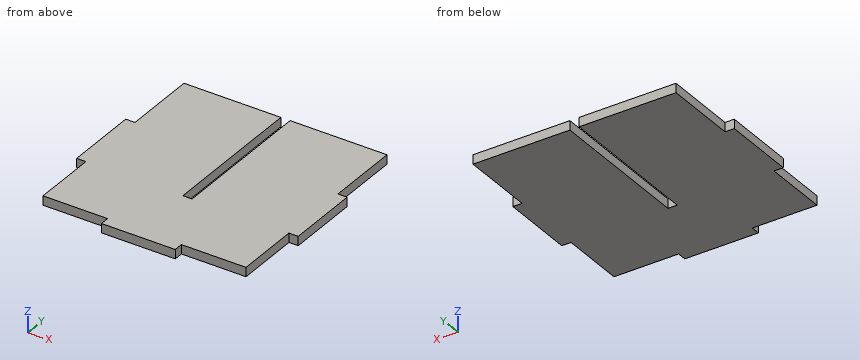
from build123d import *

# Parameters (mm, degrees)
F0_W     = 3.175
F0_H     = 25.4
F0_W_2   = 25.4
F0_H_2   = 3.175
F1_DEPTH = 3.175


with BuildPart() as f1:
    # F0 (on Top) → F1 (new body)
    with BuildSketch(Plane.XY):
        Polygon((34.925, -47.625), (34.925, -25.4), (1.5875, -25.4), (-1.5875, -25.4), (-34.925, -25.4), (-34.925, -47.625), (-12.7, -47.625), (12.7, -47.625), align=None)
        Polygon((1.5875, -25.4), (34.925, -25.4), (34.925, 0), (34.925, 25.4), (1.5875, 25.4), align=None)
        with Locations((36.5125, -12.7)):
            Rectangle(F0_W, F0_H)
        Polygon((-34.925, -25.4), (-1.5875, -25.4), (-1.5875, 25.4), (-34.925, 25.4), (-34.925, 0), align=None)
        with Locations((0, -49.2125)):
            Rectangle(F0_W_2, F0_H_2)
        with Locations((-36.5125, -12.7)):
            Rectangle(F0_W, F0_H)
    extrude(amount=F1_DEPTH)


solid = f1.part
For this review, take the finished solid that the model builds, in its own axes (mm). Give positions to 0.01 mm unless a question says otherwise; leave off trailing zeros. Loops run counter-clockwise (first coordinate to the right, second up) from the corner with the lowest first, then second, coordinate; pieces in that order, holes last. Notation, with made-up numbers: M -25.75,-35.5 L 3.25,-35.5 A11 ccw 3.25,-30.5 Z; hole C 8,-9 d8. An arc over 180 degrees is marked long. Put each result on its own line as item: value. Start each with the question number.
(1) Add section D-D, the plane x = 0. Write out the cut boundary in (y, z) (3 decimals), then the cut area to 3 significant figures.
(2) For pin 1 (1.6 mm diameter, centred on x = 36.5, z = 1.5, fed in from -Y); pin 2 (1.5 mm diameter, centred on y = 1, z = 1.5, fed in from -X) (3 decimals); pin 3 (1.6 mm diameter, centred on y = -50, z = 2.5, fed in from +X); pin 4 (1 mm diameter, centred on x = -25.5, y = -27, fed in from -Z), all flat-tipped, find the tip position at first contact; note any pin that passes through.
(3) Wall thickness on L1, parallel to X at y = 14, z = 2.05 (1 decimal); L2, parallel to X at y = -19, z = 0.5; L3, parallel to Y at x = -33, z = 0.2 (3 decimals): over which ranges is each line inside the solid? List them lowest first.
(4) Add section A-A, the plane y = -6. Write out the cut boundary in (x, z) (1 decimal), then the cut area to 3 significant figures.
(5) Add section C-C, the plane y = 3. Write out the cut boundary in (x, z) (1 decimal).
(6) Add section B-B, the plane z = 0.8. Write out the cut boundary in (x, y) (1 decimal), then the cut area to 3 significant figures.
Result:
1. outline: M -50.8,0 L -25.4,0 L -25.4,3.175 L -50.8,3.175 Z
1. area: 80.6 mm^2
2. pin 1: stops at y = -25.4
2. pin 2: stops at x = -34.925
2. pin 3: stops at x = 12.7
2. pin 4: stops at z = 0
3. L1: x = -34.9 to -1.6, 1.6 to 34.9
3. L2: x = -38.1 to -1.59, 1.59 to 38.1
3. L3: y = -47.625 to 25.4
4. outline: M -38.1,0 L -1.6,0 L -1.6,3.2 L -38.1,3.2 Z; M 1.6,0 L 38.1,0 L 38.1,3.2 L 1.6,3.2 Z
4. area: 232 mm^2
5. outline: M -34.9,0 L -1.6,0 L -1.6,3.2 L -34.9,3.2 Z; M 1.6,0 L 34.9,0 L 34.9,3.2 L 1.6,3.2 Z
6. outline: M -38.1,-25.4 L -34.9,-25.4 L -34.9,-47.6 L -12.7,-47.6 L -12.7,-50.8 L 12.7,-50.8 L 12.7,-47.6 L 34.9,-47.6 L 34.9,-25.4 L 38.1,-25.4 L 38.1,0 L 34.9,0 L 34.9,25.4 L 1.6,25.4 L 1.6,-25.4 L -1.6,-25.4 L -1.6,25.4 L -34.9,25.4 L -34.9,0 L -38.1,0 Z
6. area: 5,180 mm^2
